from build123d import *

# Parameters (mm, degrees)
BOSS_EXTRUDE1_DEPTH = 73
SKETCH2_W           = 5
SKETCH2_H           = 10
BOSS_EXTRUDE2_DEPTH = 50


with BuildPart() as part:
    # Sketch1 → Boss-Extrude1 (new body)
    with BuildSketch(Plane.XY):
        with BuildLine():
            Line((-20, -10), (20, -10))
            ThreePointArc((20, -10), (30, 0), (20, 10))
            Line((20, 10), (-20, 10))
            ThreePointArc((-20, 10), (-30, 0), (-20, -10))
        make_face()
    extrude(amount=BOSS_EXTRUDE1_DEPTH)

    # Sketch2 → Boss-Extrude2 (add)
    with BuildSketch(Plane(origin=(0, 0, 0), x_dir=(0, 0, -1), z_dir=(1, 0, 0))):
        with Locations((-2.5, 0)):
            Rectangle(SKETCH2_W, SKETCH2_H)
    extrude(amount=BOSS_EXTRUDE2_DEPTH)


solid = part.part
Could you check a few things on this model? Use its own coordinates, in mm. A direction names the side the tool comes from. Give positions to 0.01 mm unless a question says otherwise; leave off trailing zeros. Write each loop counter-clockwise with the first axis right and the second up, starting at its lowest first coordinate (ties: lowest second). Pieces come first, ordered by that corner, then holes. Notation, with made-up numbers: (28, 33.5) -> (57, 33.5) arc R13 ccw to (57, 41.5) -> close; hole circle Ø3 at (52, 10.5). An arc over 180 degrees is marked (long way). Answer as CSV lines item,"result". Start each with the question number.
(1) Which directions (+Z, -Z, +X, -X, +Y, -Y) give clear straight access to the entire face, cutting with the end or side of a thin tool? Please do faces 1 (the face through (39, 5, 3)), 2 (the face through (39, -5, 3)), 3 (the face through (0, 0, 73)).
(2) If we section it at C-C, the plane z = 12: Write out the boundary of the cut face in (x, y).
(3) If we section it at B-B, the plane x = 36: Write out the boundary of the cut face in (y, z).
(4) Please list where these lines run through material, in increasing order: line 1 (Z direction, x = 45, y = 1); line 2 (X direction, y = 1.25, z = 40.5); line 3 (X direction, y = 5.25, z = 26).
(5) If we section it at A-A, the plane y = 0: Write out the boundary of the cut face in (x, z).
(6) I'm going to push flat-ended pins straight in: pin 1 Ø5 at (x, y) = (41.5, -0.5) entering from +Z; pin 2 Ø3 at (y, z) = (-2, 58) entering from -X; pin 3 Ø4 at (x, z) = (24.5, 41.5) entering from -Y. Where does each tip first touch, or does it pass through?
Answer list:
1,face 1,"+Z, -Z, +X, +Y"
1,face 2,"+Z, -Z, +X, -Y"
1,face 3,"+Z, +X, -X, +Y, -Y"
2,outline,"(-20, -10) -> (20, -10) arc R10 ccw to (20, 10) -> (-20, 10) arc R10 ccw to start"
3,outline,"(-5, 0) -> (5, 0) -> (5, 5) -> (-5, 5) -> close"
4,line 1,"0 to 5"
4,line 2,"-29.92 to 29.92"
4,line 3,"-28.51 to 28.51"
5,outline,"(-30, 0) -> (50, 0) -> (50, 5) -> (30, 5) -> (30, 73) -> (-30, 73) -> close"
6,pin 1,"z = 5"
6,pin 2,"x = -29.99"
6,pin 3,"y = -9.68"
